Can you work these out from the model? Positions are in its coordinate system, mm. Face numbers are marked on the shaded views. A direction names the side the tool comes from. Give positions to 0.01 mm unless a question says otherwise; leave off trailing zeros. Order: outer loops, then holes, each group sorted by start corner. A loop starts at its lowest first (then second) coordinate and runs counter-clockwise, first axis right, second up. Notation, with made-up numbers: (64.5, 36.5) - (95.5, 36.5) arc R24 cw to (95.5, 67.5) - close; hole circle Ø7 at (70.5, 20). An arc over 180 degrees is marked (long way). Answer as a JSON object with one key per item and string values.
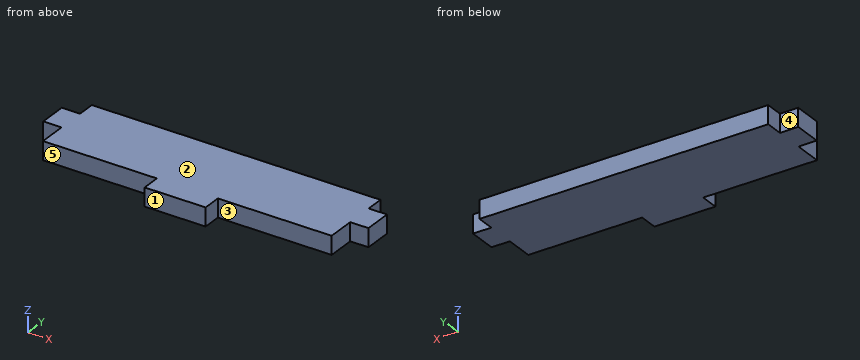
```python
from build123d import *

# Parameters (mm, degrees)
SKETCH1_W           = 9
SKETCH1_H           = 13.666666666
SKETCH1_W_2         = 30
SKETCH1_H_2         = 9
BOSS_EXTRUDE1_DEPTH = 9


with BuildPart() as part:
    # Sketch1 → Boss-Extrude1 (new body)
    with BuildSketch(Plane.XY):
        Polygon((9, 9), (65, 9), (95, 9), (151, 9), (151, 22.666666667), (151, 36.333333333), (151, 45), (9, 45), (9, 36.333333333), (9, 22.666666667), align=None)
        with Locations((4.5, 29.5)):
            Rectangle(SKETCH1_W, SKETCH1_H)
        with Locations((80, 4.5)):
            Rectangle(SKETCH1_W_2, SKETCH1_H_2)
        with Locations((155.5, 29.5)):
            Rectangle(SKETCH1_W, SKETCH1_H)
    extrude(amount=BOSS_EXTRUDE1_DEPTH)


solid = part.part
```
Q1. Which directions (+Z, -Z, +X, -X, +Y, -Y) give clear straight access to the entire face, cutting with the end or side of a thin tool? Please do the marked faces 1, 2, 3, 4 and 5.
Recorded:
{"face 1": "+Z, -Z, +X, -X, -Y", "face 2": "+Z, +X, -X, +Y, -Y", "face 3": "+Z, -Z, +X, -Y", "face 4": "+Z, -Z, -X, +Y", "face 5": "+Z, -Z, -X, -Y"}
Q2. I need wall thicknesses on L1, parallel to X at y = 7.5, z = 5; L2, parallel to Y at x = 139.5, z = 2.5; L3, parallel to X at y = 38, z = 0.5. Which ranges of each line are inside material? Lowest first, please.
Recorded:
{"L1": "x = 65 to 95", "L2": "y = 9 to 45", "L3": "x = 9 to 151"}
Q3. If we section it at A-A, the plane z = 2.5: Please give me the cut outline in (x, y).
Recorded:
{"outline": "(0, 22.67) - (9, 22.67) - (9, 9) - (65, 9) - (65, 0) - (95, 0) - (95, 9) - (151, 9) - (151, 22.67) - (160, 22.67) - (160, 36.33) - (151, 36.33) - (151, 45) - (9, 45) - (9, 36.33) - (0, 36.33) - close"}
Q4. If we section it at B-B, the plane x = 17: Please give me the cut outline in (y, z), then the cut area to 3 significant figures.
Recorded:
{"outline": "(9, 0) - (45, 0) - (45, 9) - (9, 9) - close", "area": "324 mm^2"}
Q5. If we section it at C-C, the plane y = 11: Please give me the cut outline in (x, z), then the cut area to 3 significant figures.
Recorded:
{"outline": "(9, 0) - (151, 0) - (151, 9) - (9, 9) - close", "area": "1,280 mm^2"}
Q6. I'm going to push flat-ended pins straight in: pin 1 Ø4.5 at (x, z) = (3.5, 2.5) entering from -Y; pin 2 Ø6 at (x, y) = (56, 36.5) entering from -Z; pin 3 Ø2.5 at (x, z) = (113, 4.5) entering from -Y; pin 4 Ø4 at (x, y) = (111.5, 6) entering from -Z. Where does each tip first touch, or does it pass through?
Recorded:
{"pin 1": "stops at y = 22.67", "pin 2": "stops at z = 0", "pin 3": "stops at y = 9", "pin 4": "passes through"}
